```python
from build123d import *

# Parameters (mm, degrees)
SKETCH047_W             = 182.6
SKETCH047_H             = 48
PAD017_DEPTH            = 12
SKETCH048_W             = 3
SKETCH048_H             = 48
POCKET030_DEPTH         = 9
SKETCH049_W             = 182.6
SKETCH049_H             = 3
POCKET031_DEPTH         = 3
SKETCH054_R             = 1.5
POCKET033_DEPTH         = 12
BODY015_PLACEMENT_ANGLE = 90
BODY018_PLACEMENT_ANGLE = 180


with BuildPart() as part:
    # Sketch047 → Pad017 (new body)
    with BuildSketch(Plane.XY):
        with Locations((0, 24)):
            Rectangle(SKETCH047_W, SKETCH047_H)
    extrude(amount=PAD017_DEPTH)

    # Sketch048 (on Face6 of Pad017) → Pocket030 (cut)
    with BuildSketch(Plane.XY.offset(12)):
        with Locations((-89.8, 24)):
            Rectangle(SKETCH048_W, SKETCH048_H)
    pocket030 = extrude(amount=-POCKET030_DEPTH, mode=Mode.SUBTRACT)

    # Mirrored002: Pocket030 across Sketch048 V_Axis
    add(pocket030.mirror(Plane(origin=(0, 0, 12), x_dir=(0, 0, 1), z_dir=(1, 0, 0))), mode=Mode.SUBTRACT)

    # Sketch049 (on Face2 of Mirrored002) → Pocket031 (cut)
    with BuildSketch(Plane(origin=(0, 0, 0), x_dir=(1, 0, 0), z_dir=(0, 0, -1))):
        with Locations((0, -4.5)):
            Rectangle(SKETCH049_W, SKETCH049_H)
    extrude(amount=-POCKET031_DEPTH, mode=Mode.SUBTRACT)

    # Sketch054 (on Face6 of Pocket031) → Pocket033 (cut)
    with BuildSketch(Plane.XY.offset(12)):
        with Locations((-70, 24)):
            Circle(SKETCH054_R)
    pocket033 = extrude(amount=-POCKET033_DEPTH, mode=Mode.SUBTRACT)

    # Mirrored003: Pocket033 across Sketch054 V_Axis
    add(pocket033.mirror(Plane(origin=(0, 0, 12), x_dir=(0, 0, 1), z_dir=(1, 0, 0))), mode=Mode.SUBTRACT)


with BuildPart() as part_1:
    # Body015 placement: moved
    add(part.part.moved(Location((0, 12, 0))).rotate(Axis((0, 12, 0), (1, 0, 0)), BODY015_PLACEMENT_ANGLE))


with BuildPart() as part_2:
    # Body018 placement: moved
    add(part_1.part.moved(Location((0, 206, 0))).rotate(Axis((0, 206, 0), (0, 0, 1)), BODY018_PLACEMENT_ANGLE))


solid = part_2.part
```
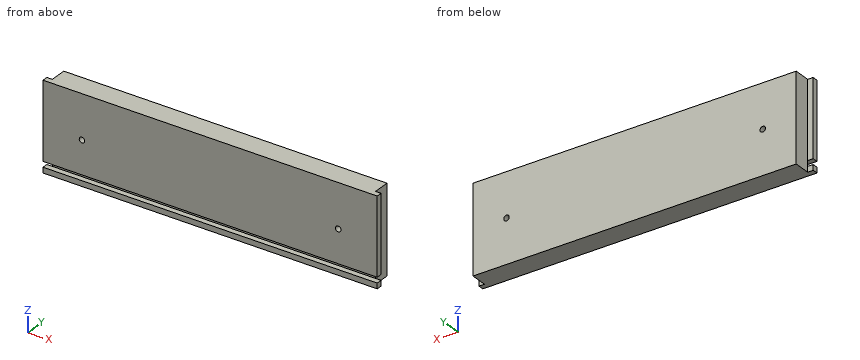
For this review, take the finished solid that the model builds, in its own axes (mm). Coordinates: 2 decimals unless noted, no trailing zeros. Write each loop counter-clockwise with the first axis right and the second up, starting at its lowest first coordinate (ties: lowest second). Pieces come first, ordered by that corner, then holes. Notation, with made-up numbers: (-5.75, 27.5) -> (28.25, 27.5) arc R31 ccw to (28.25, 53.5) -> close; hole circle Ø2 at (-16, 37). An arc over 180 degrees is marked (long way). Put each result on its own line as item: value.
Q1. Wall thickness on L1, parallel to Z at x = 35.5, y = 195.5; L2, parallel to Z at x = -70, y = 197.5; L3, parallel to X at y = 199.5, z = 32: over which ranges is each line inside the solid? List them lowest first.
From the geometry:
L1: z = 0 to 3, 6 to 48
L2: z = 0 to 22.5, 25.5 to 48
L3: x = -88.3 to 88.3
Q2. Take a section at B-B, the plane z = 33.5. State the section outline as (x, y) points, then the cut area to 3 significant figures.
From the geometry:
outline: (-91.3, 194) -> (91.3, 194) -> (91.3, 197) -> (88.3, 197) -> (88.3, 206) -> (-88.3, 206) -> (-88.3, 197) -> (-91.3, 197) -> close
area: 2,140 mm2
Q3. Take a section at C-C, the plane y = 201.25. State the section outline as (x, z) points, then the cut area to 3 significant figures.
From the geometry:
outline: (-88.3, 0) -> (88.3, 0) -> (88.3, 48) -> (-88.3, 48) -> close; hole circle Ø3 at (-70, 24); hole circle Ø3 at (70, 24)
area: 8,460 mm2
Q4. Take a section at A-A, the plane x = 44. State the section outline as (y, z) points.
From the geometry:
outline: (194, 0) -> (206, 0) -> (206, 48) -> (194, 48) -> (194, 6) -> (197, 6) -> (197, 3) -> (194, 3) -> close
Q5. Clearance check with flat-ended pins moving along their axes: pin 1 Ø0.9 at (x, z) = (-89.5, 2) entering from +Y; pin 2 Ø2.5 at (y, z) = (203.5, 13) entering from -X; pin 3 Ø4.5 at (y, z) = (199.5, 20) entering from +X; pin 4 Ø2.5 at (x, z) = (-70, 24) entering from +Y. State where each tip first meets the part, or that it passes through.
From the geometry:
pin 1: stops at y = 197
pin 2: stops at x = -88.3
pin 3: stops at x = 88.3
pin 4: passes through
